Build history of the part. All positions in model axes, mm. A direction names the side the tool comes from. Give positions to 0.01 mm unless a question says otherwise; leave off trailing zeros. Loops run counter-clockwise (first coordinate to the right, second up) from the corner with the lowest first, then second, coordinate; pieces in that order, holes last. Notation, with made-up numbers: M 59,14.5 L 66,14.5 A32 cw 66,42.5 Z; hole C -2,48 d11. An arc over 180 degrees is marked long. Answer as a JSON object with one key per item and string values. Group by question number.
1. Slice it at B-B (x = 104). List the corners of the cut face in (y, z).
2. 3-axis set-ups, long thin cutter, end or side, ignore diameter. For faces 1 (the face through (64, 6.028, -20)), 2 (the face through (135.506, 14.301, 92.308)), 3 (the face through (128, 6, 73.025)), 4 (the face through (-3.175, 16, 68)), 5 (the face through (136, 5, 111.125)): which of +Z, -Z, +X, -X, +Y, -Y reach the whole face in a straight line?
3. Drill centre lines: line 1 along Z through (x, y) = (132.5, 8.75) (3 decimals); line 2 along X through (y, z) = (7, 8); line 3 along Z through (x, y) = (38, 8.25). Where is each one in solid material? Low to high. Write a range as [from, to].
4. Drop flat-ended pins along their axis: pin 1 Ø1.6 at (y, z) = (8, -10.5) entering from -X; pin 2 Ø1 at (x, z) = (21.5, -4) entering from +Y; pin 3 Ø10 at (x, y) = (51.5, 5.5) entering from -Z; pin 4 Ø6 at (x, z) = (35, 119) entering from -Y. Give the stop position or say it passes through.
5. Mould opens along Y. For faces 6 (the face through (124.46, 10, 64)), 7 (the face through (65.56, 12.13, 128.83)), 8 (the face through (64, 9.203, -20)), 9 (the face through (63.596, 13.847, -8.072)) say: released by +Y, released by -Y, zero draft, split by the parting line, or undercut.
from build123d import *

# Parameters (mm, degrees)
BOSS_EXTRUDE1_DEPTH = 15.875
CUT_EXTRUDE1_DEPTH  = 195.237355702
BOSS_EXTRUDE2_DEPTH = 6.35
FILLET1_R           = 1.27
BOSS_EXTRUDE3_DEPTH = 7.9375
SKETCH5_W           = 12.7
SKETCH5_H           = 3.175
BOSS_EXTRUDE4_DEPTH = 40.9575


with BuildPart() as part:
    # Sketch1 → Boss-Extrude1 (new body)
    with BuildSketch(Plane(origin=(0, 0, 0), x_dir=(1, 0, 0), z_dir=(0, 1, 0))):
        Polygon((0, 0), (137.16, 0), (137.16, -53.975), (124.46, -53.975), (124.46, -73.025), (130.81, -73.025), (130.81, -92.075), (140.335, -92.075), (140.335, -111.125), (132.3975, -111.125), (132.3975, -133.35), (0, -133.35), align=None)
    extrude(amount=BOSS_EXTRUDE1_DEPTH)

    # Sketch2 → Cut-Extrude1 (cut, through all)
    with BuildSketch(Plane.ZY):
        Polygon((133.35, 7.9375), (133.35, 15.875), (0, 15.875), align=None)
    extrude(amount=-CUT_EXTRUDE1_DEPTH, mode=Mode.SUBTRACT)

    # Sketch3 → Boss-Extrude2 (add)
    with BuildSketch(Plane(origin=(0, 15.818952125, 0.941604293), x_dir=(1, 0, 0), z_dir=(0, 0.9982331517348171, 0.05941863998421531))):
        Polygon((-7.9375, 8.88077091), (137.16, 8.88077091), (137.16, -6.99422909), (7.9375, -6.99422909), (7.9375, -124.705255329), (132.3975, -124.705255329), (132.3975, -140.580255329), (-7.9375, -140.580255329), align=None)
    extrude(amount=-BOSS_EXTRUDE2_DEPTH)

    # Fillet1
    fillet1_edges = [part.edges().sort_by_distance(p)[0] for p in [
        (-7.9375, 5.567469486, 66.297691636),
        (64.61125, 10.007854941, -8.300784006),
        (62.23, 1.127084032, 140.896167278),
    ]]
    fillet(fillet1_edges, radius=FILLET1_R)

    # Sketch4 → Boss-Extrude3 (add)
    with BuildSketch(Plane(origin=(0, 15.818952125, 0.941604293), x_dir=(1, 0, 0), z_dir=(0, 0.9982331517348171, 0.05941863998421531))):
        Polygon((-3.175, -3.81922909), (103.849852773, -3.81922909), (137.16, -3.81922909), (137.16, -53.12726352), (124.46, -53.12726352), (124.46, -72.210981554), (130.81, -72.210981554), (130.81, -91.294699588), (140.335, -91.294699588), (140.335, -110.378417623), (132.3975, -110.378417623), (132.3975, -127.880255329), (-3.175, -127.880255329), align=None)
    extrude(amount=BOSS_EXTRUDE3_DEPTH)

    # Sketch5 → Boss-Extrude4 (add)
    with BuildSketch(Plane(origin=(0, 0, 0), x_dir=(-1, 0, 0), z_dir=(0, 0, -1))):
        with Locations((-63.5, 7.615385455)):
            Rectangle(SKETCH5_W, SKETCH5_H)
        with Locations((-105.41, 7.615385455)):
            Rectangle(SKETCH5_W, SKETCH5_H)
    extrude(amount=BOSS_EXTRUDE4_DEPTH)


solid = part.part
Established:
{
 "1": {"outline": "M 0,0 L 6.03,0 L 6.03,-40.96 L 9.2,-40.96 L 9.2,0 L 9.51,0 L 9.93,-7.03 A1.27 ccw 11.28,-8.23 L 16.35,-7.92 L 15.59,4.75 L 23.52,5.23 L 16.14,129.07 L 8.22,128.6 L 7.47,141.27 L 2.39,140.97 A1.27 ccw 1.2,139.63 L 1.58,133.35 L 0,133.35 Z"},
 "2": {"face 1": "-Z, +X, -X, -Y", "face 2": "+X, +Y", "face 3": "+X, +Y, -Y", "face 4": "+Z, -X, +Y", "face 5": "+Z, +X, -Y"},
 "3": {"line 1": "z = [0, 53.975], [92.075, 111.125]", "line 2": "x = [0, 137.16]", "line 3": "z = [0, 128.6]"},
 "4": {"pin 1": "stops at x = 57.15", "pin 2": "stops at y = 16.14", "pin 3": "stops at z = -8.02", "pin 4": "stops at y = 0"},
 "5": {"face 6": "zero draft", "face 7": "undercut", "face 8": "undercut", "face 9": "released by +Y"}
}
